Verification items for the finished model (mm, model axes). Give positions to 0.01 mm unless a question says otherwise; leave off trailing zeros. Loops run counter-clockwise (first coordinate to the right, second up) from the corner with the lowest first, then second, coordinate; pieces in that order, holes last. Notation, with made-up numbers: M -13,60.25 L 24,60.25 A17 cw 24,72.25 Z; hole C 88,-29.5 d4. An arc over 180 degrees is marked long. Use a Markdown table: item, result.
from build123d import *

# Parameters (mm, degrees)
SKETCH_1_W          = 80
SKETCH_1_H          = 110
SKETCH_1_R          = 1.5
EXTRUDE_1_DEPTH     = 2
CUT_EXTRUDE_1_DEPTH = 10
FILLET_1_R          = 4


with BuildPart() as part:
    # 草图1 → 凸台-拉伸1 (new body)
    with BuildSketch(Plane.XY):
        with Locations((40, 55)):
            Rectangle(SKETCH_1_W, SKETCH_1_H)
        with Locations((10, 3)):
            Circle(SKETCH_1_R, mode=Mode.SUBTRACT)
        with Locations((30, 3)):
            Circle(SKETCH_1_R, mode=Mode.SUBTRACT)
        with Locations(Location((50, 3, 0), (0, 0, 180))):
            Circle(SKETCH_1_R, mode=Mode.SUBTRACT)
        with Locations(Location((70, 3, 0), (0, 0, 180))):
            Circle(SKETCH_1_R, mode=Mode.SUBTRACT)
        with Locations((2.5, 107)):
            Circle(SKETCH_1_R, mode=Mode.SUBTRACT)
        with Locations((2.5, 85)):
            Circle(SKETCH_1_R, mode=Mode.SUBTRACT)
        with Locations(Location((77.5, 85, 0), (0, 0, 180))):
            Circle(SKETCH_1_R, mode=Mode.SUBTRACT)
        with Locations(Location((77.5, 107, 0), (0, 0, 180))):
            Circle(SKETCH_1_R, mode=Mode.SUBTRACT)
        with Locations((10, 27)):
            Circle(SKETCH_1_R, mode=Mode.SUBTRACT)
        with Locations((30, 27)):
            Circle(SKETCH_1_R, mode=Mode.SUBTRACT)
        with Locations(Location((50, 27, 0), (0, 0, 180))):
            Circle(SKETCH_1_R, mode=Mode.SUBTRACT)
        with Locations(Location((70, 27, 0), (0, 0, 180))):
            Circle(SKETCH_1_R, mode=Mode.SUBTRACT)
    extrude(amount=EXTRUDE_1_DEPTH)

    # 草图3 → 切除-拉伸1 (cut)
    with BuildSketch(Plane.XY.offset(2)):
        Polygon((10, 100), (10, 35), (57.604900254, 35), align=None)
        Polygon((22.395099746, 100), (70, 35), (70, 100), align=None)
    extrude(amount=-CUT_EXTRUDE_1_DEPTH, mode=Mode.SUBTRACT)

    # 圆角1
    fillet_1_edges = [part.edges().sort_by_distance(p)[0] for p in [
        (22.395099746, 100, 1),
        (70, 100, 1),
        (70, 35, 1),
        (10, 100, 1),
        (57.604900254, 35, 1),
        (10, 35, 1),
    ]]
    fillet(fillet_1_edges, radius=FILLET_1_R)


solid = part.part
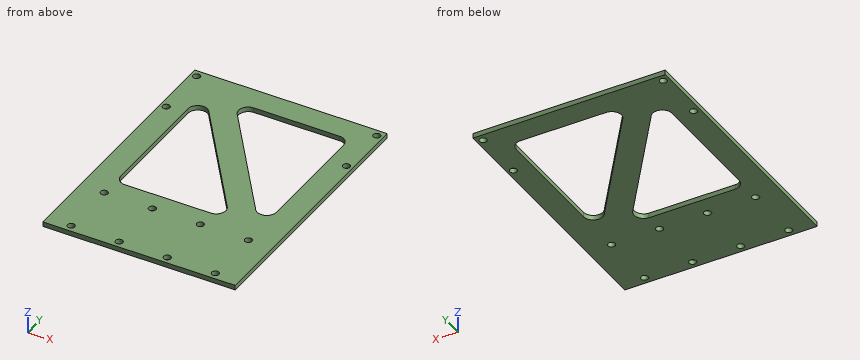
(1) Cross-section at B-B on z = 1.1. State how many separate pieces and enclosed holes the cut face has, then the cut area to 3 significant figures.
Results below:
| item | result |
|---|---|
| separate pieces | 1 |
| enclosed holes | 14 |
| area | 5,710 mm^2 |
(2) Material ranges on line 1 (Y direction, x = 2.5, z = 1.3); line 2 (X direction, y = 107, z = 1.1); line 3 (X direction, y = 85, z = 0.75), recorded low to high.
Results below:
| item | result |
|---|---|
| line 1 | 0 to 83.5, 86.5 to 105.5, 108.5 to 110 |
| line 2 | 0 to 1, 4 to 76, 79 to 80 |
| line 3 | 0 to 1, 4 to 10, 20.99 to 33.38, 70 to 76, 79 to 80 |
(3) Cross-section at A-A on x = 77.5. Record the cut outline in (y, z).
Results below:
| item | result |
|---|---|
| outline | M 0,0 L 83.5,0 L 83.5,2 L 0,2 Z; M 86.5,0 L 105.5,0 L 105.5,2 L 86.5,2 Z; M 108.5,0 L 110,0 L 110,2 L 108.5,2 Z |
(4) Cross-section at C-C on y = 107. Record the cut outline in (x, z), then the cut area to 3 significant figures.
Results below:
| item | result |
|---|---|
| outline | M 0,0 L 1,0 L 1,2 L 0,2 Z; M 4,0 L 76,0 L 76,2 L 4,2 Z; M 79,0 L 80,0 L 80,2 L 79,2 Z |
| area | 148 mm^2 |
(5) Gauge pin test, flat end, axial feed: P1, Ø2.5, axis at x = 10, y = 27, coming from the +Z side. Record the tip position at first contact, or that the pin passes through.
Results below:
| item | result |
|---|---|
| P1 | through |
